Geometry check sheet. Reference: the model listing, model coordinates, mm. A direction names the side the tool comes from. Coordinates: 2 decimals unless noted, no trailing zeros. Loops run counter-clockwise (first coordinate to the right, second up) from the corner with the lowest first, then second, coordinate; pieces in that order, holes last. Notation, with made-up numbers: (28, 35.25) -> (38, 35.25) arc R25 cw to (38, 63.25) -> close; hole circle Ø9 at (-30.5, 46). An arc over 180 degrees is marked (long way). Answer as a JSON object with one key per item and string values.
from build123d import *

# Parameters (mm, degrees)
SKETCH1_R           = 30.48
SKETCH1_W           = 7.874
SKETCH1_H           = 8.128
BOSS_EXTRUDE1_DEPTH = 12.7


with BuildPart() as part:
    # Sketch1 → Boss-Extrude1 (new body)
    # profile 1 of 2: a face of its own
    with BuildSketch(Plane.XY):
        Circle(SKETCH1_R)
        with BuildLine():
            Line((-3.937, 17.078076795), (-3.937, 21.59))
            Line((-3.937, 21.59), (3.937, 21.59))
            Line((3.937, 21.59), (3.937, 17.078076795))
            ThreePointArc((3.937, 17.078076795), (0, -17.526), (-3.937, 17.078076795))
        make_face(mode=Mode.SUBTRACT)
    # profile 2 of 2: a face of its own
    with BuildSketch(Plane.XY):
        with Locations((0, 17.526)):
            Rectangle(SKETCH1_W, SKETCH1_H)
    extrude(amount=BOSS_EXTRUDE1_DEPTH)


solid = part.part
1. Section check B-B, the plane y = 0. Record the boundary of the cut face in (x, z), then the cut area to 3 significant figures.
Evaluation:
{"outline": "(-30.48, 0) -> (-17.53, 0) -> (-17.53, 12.7) -> (-30.48, 12.7) -> close; (17.53, 0) -> (30.48, 0) -> (30.48, 12.7) -> (17.53, 12.7) -> close", "area": "329 mm^2"}
2. Thickness scan on probe 1 along Y at (x, z) = (0, 4); probe 2 along X at (y, z) = (-6, 8); probe 3 along Y at (x, z) = (-5, 10). Record the ranges inside material, lowest first. Write a range as from..to.
Evaluation:
{"probe 1": "y = -30.48..-17.53, 13.46..30.48", "probe 2": "x = -29.88..-16.47, 16.47..29.88", "probe 3": "y = -30.07..-16.8, 16.8..30.07"}
3. Section check C-C, the plane z = 3. Record the boundary of the cut face in (x, y).
Evaluation:
{"outline": "circle Ø60.96 at (0, 0); hole (-3.94, 13.46) -> (-3.94, 17.08) arc R17.53 ccw (long way) to (3.94, 17.08) -> (3.94, 13.46) -> close"}
4. Section check A-A, the plane x = 0. Record the boundary of the cut face in (y, z), then the cut area to 3 significant figures.
Evaluation:
{"outline": "(-30.48, 0) -> (-17.53, 0) -> (-17.53, 12.7) -> (-30.48, 12.7) -> close; (13.46, 0) -> (30.48, 0) -> (30.48, 12.7) -> (13.46, 12.7) -> close", "area": "381 mm^2"}
5. Mould release check, pull along Y, two halves, no side actions. Record for faces 3 (the face through (-6.607, -29.755, 6.261)), 4 (the face through (0, 14, 12.7)), 5 (the face through (0.72, -17.51, 6.26)): released by +Y, released by -Y, zero draft, split by the parting line, or undercut.
Evaluation:
{"face 3": "split by the parting line", "face 4": "zero draft", "face 5": "undercut"}
6. Tool access check on faces 1 (the face through (0, 14, 0)), 2 (the face through (0, 13.462, 6)). Record the directions out of +Z, -Z, +X, -X, +Y, -Y that give a thin tool (end or side, any length) a straight path to the whole face; none if there is none.
Evaluation:
{"face 1": "-Z, +X, -X, +Y, -Y", "face 2": "+Z, -Z"}
7. Depth check by flat-ended pin: P1, Ø1.8, axis at y = 16, z = 7.5, coming from the +X side; P2, Ø4, axis at x = -2, z = 4, coming from the -Y side; P3, Ø3, axis at y = -18.5, z = 6, coming from the +X side; P4, Ø1.5, axis at x = 15.5, y = 4, coming from the +Z side. Enter the tip coordinate at first touch or a pass-through.
Evaluation:
{"P1": "stops at x = 26.48", "P2": "stops at y = -30.48", "P3": "stops at x = 25.3", "P4": "passes through"}
8. Section check D-D, the plane y = -25. Record the boundary of the cut face in (x, z).
Evaluation:
{"outline": "(-17.44, 0) -> (17.44, 0) -> (17.44, 12.7) -> (-17.44, 12.7) -> close"}
